from build123d import *

# Parameters (mm, degrees)
SKETCH1_W           = 7.3
SKETCH1_H           = 8
BOSS_EXTRUDE1_DEPTH = 5
SKETCH1_3_W         = 7.3
SKETCH1_3_H         = 8
BOSS_EXTRUDE2_DEPTH = 1
BOSS_EXTRUDE3_DEPTH = 3
CHAMFER1_SIZE       = 1
FILLET1_R           = 0.5


with BuildPart() as part:
    # Sketch1 → Boss-Extrude1 (new body)
    with BuildSketch(Plane.XY):
        Rectangle(SKETCH1_W, SKETCH1_H)
        with BuildLine():
            Line((-1.183215957, 1.15), (1.183215957, 1.15))
            ThreePointArc((1.183215957, 1.15), (0, -1.65), (-1.183215957, 1.15))
        make_face(mode=Mode.SUBTRACT)
    extrude(amount=BOSS_EXTRUDE1_DEPTH)

    # Sketch1<3> → Boss-Extrude2 (add)
    with BuildSketch(Plane.XY):
        Rectangle(SKETCH1_3_W, SKETCH1_3_H)
    extrude(amount=-BOSS_EXTRUDE2_DEPTH)

    # Sketch2 → Boss-Extrude3 (add)
    with BuildSketch(Plane(origin=(0, 0, -1), x_dir=(-1, 0, 0), z_dir=(0, 0, -1))):
        with BuildLine():
            Line((3.65, -4), (3.65, 4))
            Line((3.65, 4), (-10.35, 4))
            ThreePointArc((-10.35, 4), (-11.35, 3), (-12.35, 4))
            Line((-12.35, 4), (-14.35, 4))
            Line((-14.35, 4), (-14.35, -4))
            Line((-14.35, -4), (-12.35, -4))
            ThreePointArc((-12.35, -4), (-11.35, -3), (-10.35, -4))
            Line((-10.35, -4), (3.65, -4))
        make_face()
    extrude(amount=BOSS_EXTRUDE3_DEPTH)

    # Chamfer1
    chamfer1_edges = [part.edges().sort_by_distance(p)[0] for p in [
        (-3.65, 0, -4),
    ]]
    chamfer(chamfer1_edges, length=CHAMFER1_SIZE)

    # Fillet1
    fillet1_edges = [part.edges().sort_by_distance(p)[0] for p in [
        (-3.65, -4, 1),
        (-3.65, 4, 1),
        (3.65, 4, 2),
        (3.65, -4, 2),
        (0, -4, 5),
        (3.65, 0, 5),
        (0, 4, 5),
        (3.65, 0, -1),
        (-3.65, 0, 5),
        (7, 4, -1),
        (11.35, 3, -1),
        (13.35, 4, -1),
        (14.35, 0, -1),
        (14.35, 4, -2.5),
        (14.35, -4, -2.5),
        (7, -4, -1),
        (11.35, -3, -1),
        (13.35, -4, -1),
        (0, 1.15, 5),
        (0, -1.65, 5),
    ]]
    fillet(fillet1_edges, radius=FILLET1_R)


solid = part.part
Design review of the part built by this model. Coordinates are the model's own, in mm. A direction names the side the tool comes from. Give positions to 0.01 mm unless a question says otherwise; leave off trailing zeros. Order: outer loops, then holes, each group sorted by start corner. A loop starts at its lowest first (then second) coordinate and runs counter-clockwise, first axis right, second up.
1. Add section B-B, the plane x = 0. State the section outline as (y, z) points, then the cut area to 3 significant figures.
Solution:
outline: (-4, -4) - (4, -4) - (4, 4.5) arc R0.5 ccw to (3.5, 5) - (1.65, 5) arc R0.5 ccw to (1.15, 4.5) - (1.15, 0) - (-1.65, 0) - (-1.65, 4.5) arc R0.5 ccw to (-2.15, 5) - (-3.5, 5) arc R0.5 ccw to (-4, 4.5) - close
area: 57.8 mm2
2. Tool access review of faces 1 (the flat face through (9, 0, -1)), 2 (the cylindrical face through (0.05, -1.65, 2.22)), 3 (the flat face through (14.35, 0, -3)): name each direction out of +Z, -Z, +X, -X, +Y, -Y from which nothing blocks a thin tool from reaching the whole face with its end or side.
Solution:
face 1: +Z, +X, +Y, -Y
face 2: +Z
face 3: +Z, -Z, +X, +Y, -Y
3. Add section A-A, the plane z = 1.25. State the section outline as (x, y) points, then the cut area to 3 significant figures.
Solution:
outline: (-3.65, -3.5) arc R0.5 ccw to (-3.15, -4) - (3.15, -4) arc R0.5 ccw to (3.65, -3.5) - (3.65, 3.5) arc R0.5 ccw to (3.15, 4) - (-3.15, 4) arc R0.5 ccw to (-3.65, 3.5) - close; hole (-1.18, 1.15) arc R1.65 ccw (long way) to (1.18, 1.15) - close
area: 50.4 mm2
4. Add section C-C, the plane z = -1.75. State the section outline as (x, y) points, then the cut area to 3 significant figures.
Solution:
outline: (-3.65, -3.5) arc R0.5 ccw to (-3.15, -4) - (10.35, -4) arc R1 cw to (12.35, -4) - (13.85, -4) arc R0.5 ccw to (14.35, -3.5) - (14.35, 3.5) arc R0.5 ccw to (13.85, 4) - (12.35, 4) arc R1 cw to (10.35, 4) - (-3.15, 4) arc R0.5 ccw to (-3.65, 3.5) - close
area: 141 mm2
5. Mouldability with a two-part tool opening along X and no side actions: class faces 4 (the flat face through (3.65, 0, 2)), 5 (the flat face through (0, 0, 0)), 6 (the flat face through (13, -4, -3)) as +X half, -X half, draft (parallel to the pull), parting line (faces both ways), or undercut.
Solution:
face 4: +X half
face 5: undercut
face 6: draft
6. For pin 1 Ø3.5 at (x, y) = (6.5, 0.5) entering from +Z; pin 2 Ø2 at (x, y) = (0.5, 0) entering from +Z; pin 3 Ø5 at (x, z) = (3.5, -0.5) entering from +Y, all flat-tipped, find the tip position at first contact; note any pin that passes through.
Solution:
pin 1: stops at z = -1
pin 2: stops at z = 0
pin 3: stops at y = 4
7. To check wall thickness, follow L1, parallel to Y at x = 0, z = 3.5; L2, parallel to X at y = 0, z = 3.2; L3, parallel to Z at x = 8, y = -1.5. State the ranges of each line that lie inside material, in increasing order.
Solution:
L1: y = -4 to -1.65, 1.15 to 4
L2: x = -3.65 to -1.65, 1.65 to 3.65
L3: z = -4 to -1
8. Add section D-D, the plane x = 9.5. State the section outline as (y, z) points.
Solution:
outline: (-4, -4) - (4, -4) - (4, -1.5) arc R0.5 ccw to (3.5, -1) - (-3.5, -1) arc R0.5 ccw to (-4, -1.5) - close
